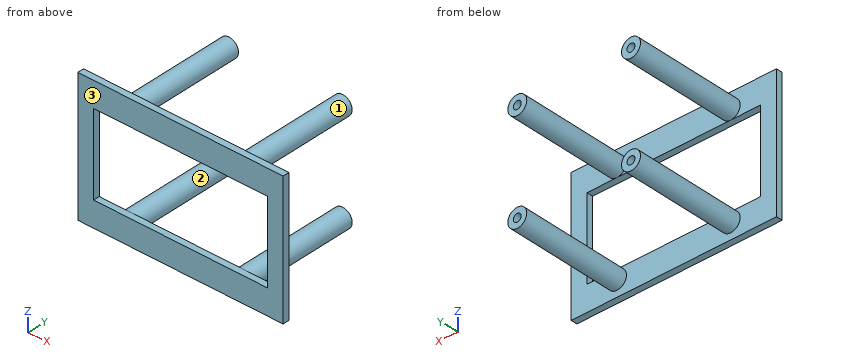
from build123d import *

# Parameters (mm, degrees)
SKETCH1_W           = 65
SKETCH1_H           = 42
SKETCH1_W_2         = 55
SKETCH1_H_2         = 26
BOSS_EXTRUDE2_DEPTH = 2
SKETCH1_3_R         = 3
SKETCH1_3_R_2       = 1.25
BOSS_EXTRUDE3_DEPTH = 35
CUT_EXTRUDE1_START  = 35
SKETCH1_4_R         = 1.25
CUT_EXTRUDE1_DEPTH  = 11


with BuildPart() as part:
    # Sketch1 → Boss-Extrude2 (new body)
    with BuildSketch(Plane(origin=(0, 0, 0), x_dir=(1, 0, 0), z_dir=(0, 1, 0))):
        Rectangle(SKETCH1_W, SKETCH1_H)
        Rectangle(SKETCH1_W_2, SKETCH1_H_2, mode=Mode.SUBTRACT)
    extrude(amount=-BOSS_EXTRUDE2_DEPTH)

    # Sketch1<3> → Boss-Extrude3 (add)
    with BuildSketch(Plane(origin=(0, 0, 0), x_dir=(1, 0, 0), z_dir=(0, 1, 0))):
        with Locations(Location((-18, 16, 0), (0, 0, 270))):
            Circle(SKETCH1_3_R)
        with Locations((-18, 16)):
            Circle(SKETCH1_3_R_2, mode=Mode.SUBTRACT)
        with Locations((-18, 16)):
            Circle(SKETCH1_3_R_2)
        with Locations(Location((18, 16, 0), (0, 0, 270))):
            Circle(SKETCH1_3_R)
        with Locations((18, 16)):
            Circle(SKETCH1_3_R_2, mode=Mode.SUBTRACT)
        with Locations((18, 16)):
            Circle(SKETCH1_3_R_2)
        with Locations(Location((18, -16, 0), (0, 0, 90))):
            Circle(SKETCH1_3_R)
        with Locations((18, -16)):
            Circle(SKETCH1_3_R_2, mode=Mode.SUBTRACT)
        with Locations(Location((-18, -16, 0), (0, 0, 90))):
            Circle(SKETCH1_3_R)
        with Locations((-18, -16)):
            Circle(SKETCH1_3_R_2, mode=Mode.SUBTRACT)
        with Locations((-18, -16)):
            Circle(SKETCH1_3_R_2)
        with Locations((18, -16)):
            Circle(SKETCH1_3_R_2)
    extrude(amount=BOSS_EXTRUDE3_DEPTH)

    # Sketch1<4> → Cut-Extrude1 (cut)
    with BuildSketch(Plane(origin=(0, 0, 0), x_dir=(1, 0, 0), z_dir=(0, 1, 0)).offset(CUT_EXTRUDE1_START)):
        with Locations(Location((-18, 16, 0), (0, 0, 270))):
            Circle(SKETCH1_4_R)
        with Locations(Location((18, 16, 0), (0, 0, 270))):
            Circle(SKETCH1_4_R)
        with Locations(Location((18, -16, 0), (0, 0, 270))):
            Circle(SKETCH1_4_R)
        with Locations(Location((-18, -16, 0), (0, 0, 270))):
            Circle(SKETCH1_4_R)
    extrude(amount=-CUT_EXTRUDE1_DEPTH, mode=Mode.SUBTRACT)


solid = part.part
Input: part model. Units: mm. Frame: model coordinates. Face numbers are marked on the shaded views. Coordinates: 2 decimals unless noted, no trailing zeros. Loops run counter-clockwise (first coordinate to the right, second up) from the corner with the lowest first, then second, coordinate; pieces in that order, holes last. Notation, with made-up numbers: (1.25, -18) - (37.25, -18) arc R14 ccw to (37.25, -1) - close; hole circle Ø3 at (76.5, 47). An arc over 180 degrees is marked (long way). Answer in a Markdown table with one row per item. Add a question column.
Item 1: Mould query, pull axis Z, two halves, no side actions, for the marked faces 1, 2 and 3. Classes: released by +Z, released by -Z, zero draft, split by the parting line, or undercut.
Item 2: Section query C-C on z = 8.5. Return the cut outline in (x, y).
Item 3: Section query A-A on y = 30. Return the cut outline in (x, z).
Item 4: Contact query for flat-ended pins moving along their axis: P1, Ø12, axis at y = 7.5, z = 14, coming from the -X side; P2, Ø1.2, axis at x = -18, z = 16, coming from the +Y side; P3, Ø4, axis at x = -17.5, y = 6.5, coming from the +Z side. Output: stop coordinate, or through.
Item 5: Section query D-D on z = 16. Return the cut outline in (x, y).
Item 6: Line query: line 1 along X through (y, z) = (26, 16); line 2 along Z through (x, y) = (18.5, 25.5); line 3 along X through (y, z) = (7, 15.5). Output: solid intervals per line, ascending. Write a range as [from, to].
Item 7: Section query B-B on x = 2. Return the cut outline in (y, z).
Recorded:
| question | item | result |
|---|---|---|
| 1 | face 1 | undercut |
| 1 | face 2 | undercut |
| 1 | face 3 | zero draft |
| 2 | outline | (-32.5, -2) - (-27.5, -2) - (-27.5, 0) - (-32.5, 0) - close; (27.5, -2) - (32.5, -2) - (32.5, 0) - (27.5, 0) - close |
| 3 | outline | circle Ø6 at (-18, -16); circle Ø6 at (-18, 16); circle Ø6 at (18, -16); circle Ø6 at (18, 16); hole circle Ø2.5 at (-18, -16); hole circle Ø2.5 at (-18, 16); hole circle Ø2.5 at (18, -16); hole circle Ø2.5 at (18, 16) |
| 4 | P1 | x = -21 |
| 4 | P2 | y = 24 |
| 4 | P3 | z = 19 |
| 5 | outline | (-32.5, -2) - (32.5, -2) - (32.5, 0) - (21, 0) - (21, 35) - (19.25, 35) - (19.25, 24) - (16.75, 24) - (16.75, 35) - (15, 35) - (15, 0) - (-15, 0) - (-15, 35) - (-16.75, 35) - (-16.75, 24) - (-19.25, 24) - (-19.25, 35) - (-21, 35) - (-21, 0) - (-32.5, 0) - close |
| 6 | line 1 | [-21, -19.25], [-16.75, -15], [15, 16.75], [19.25, 21] |
| 6 | line 2 | [-18.96, -17.15], [-14.85, -13.04], [13.04, 14.85], [17.15, 18.96] |
| 6 | line 3 | [-20.96, -15.04], [15.04, 20.96] |
| 7 | outline | (-2, -21) - (0, -21) - (0, -13) - (-2, -13) - close; (-2, 13) - (0, 13) - (0, 21) - (-2, 21) - close |
